Autodesk Inventor part; units mm, degrees
ref_plane "YZ Plane" through (0, 0, 0) normal (1, 0, 0) x (0, 1, 0)
ref_plane "XZ Plane" through (0, 0, 0) normal (0, 1, 0) x (-1, 0, 0)
ref_plane "XY Plane" through (0, 0, 0) normal (0, 0, 1) x (1, 0, 0)
sketch "Sketch1" plane through (0, 0, 0) normal (0, 0, 1) x (1, 0, 0)
  circle A0 centre (0, 0) radius 558
  circle A1 centre (0, 0) radius 580
  line L0 (0, 0) -> (-580, 0)
  line L1 (0, 0) -> (0, 580) construction
  line L2 (0, 0) -> (0, 580)
  circle A2 centre (0, 0) radius 100
  line L3 (197.082, 197.082) -> (278.716, 0)
  line L4 (278.716, 0) -> (197.082, -197.082)
  line L5 (197.082, -197.082) -> (0, -278.716)
  line L6 (0, -278.716) -> (-197.082, -197.082)
  line L7 (-197.082, -197.082) -> (-278.716, 0)
  line L8 (-278.716, 0) -> (-197.082, 197.082)
  line L9 (-197.082, 197.082) -> (0, 278.716)
  line L10 (0, 278.716) -> (197.082, 197.082)
  point P0 (-558, 0)
  point P1 (0, 558)
  point P2 (-100, 0)
  point P3 (0, 100)
  point P4 (0, 278.716)
  point P5 (-278.716, 0)
  dimension "d30" = 90
  dimension "d31" = 1160
  dimension "d32" = 1116
  dimension "d65" = 90
  dimension "d66" = 200
  dimension "d91" = 515
extrude "Plate1" add sketch "Sketch1" against normal blind 3 contours A0 L0 A1 L2 picked at (-572.0249, 22.0563)
sketch "Sketch2" plane through (0, 0, 0) normal (0, 0, 1) x (1, 0, 0)
  circle A0 centre (0, 0) radius 567.5
  arc A1 (0, 580) -> (-580, 0) centre (0, 0) ccw
  line L0 (0, 0) -> (0, 580) construction
  line L1 (0, 0) -> (-18.5681, 567.1962) construction
  line L2 (-128.8658, 552.6752) -> (0, 0) construction
  line L3 (0, 0) -> (0, 567.5) construction
  line L4 (0, 0) -> (18.5681, 567.1962) construction
  line L5 (0, 0) -> (128.8658, 552.6752) construction
  line L6 (0, 0) -> (-164.7366, 543.0636) construction
  line L7 (0, 0) -> (-267.5176, 500.4903) construction
  dimension "d34" = 1135
  dimension "d35" = 1.875
  dimension "d36" = 11.25
  dimension "d44" = 1.875
  dimension "d45" = 11.25
  dimension "d49" = 3.75
  dimension "d50" = 11.25
hole "Hole1" at (-18.5681, 567.1962, 0) at (-128.8658, 552.6752, 0) at (128.8658, 552.6752, 0) at (18.5681, 567.1962, 0) at (-164.7366, 543.0636, 0) at (-267.5176, 500.4903, 0) direction (0, 0, -1) diameter 8 end through all
pattern_circular "Circular Pattern1" count 4 over 90 about axis through (0, 0, -10) along (0, 0, 1) of "Hole1"
equation "\"d31\" = Колесо_диам1_ручья_внеш"
equation "\"d91\" = Барабан_размер_по_плоскостям"
equation "\"d44\" = d35"
equation "\"d45\" = d36"
equation "\"d49\" = 2 * d35"
equation "\"d50\" = d36"
equation "\"d42\" = Thickness"
equation "\"d15\" = Thickness"
equation "\"BendRadius\" = Thickness"
equation "\"BendReliefWidth\" = Thickness"
equation "\"BendReliefDepth\" = 0.5 * Thickness"
equation "\"CornerReliefSize\" = 4 * Thickness"
equation "\"MinimumRemnant\" = 2 * Thickness"
equation "\"TransitionRadius\" = BendRadius"
equation "\"JacobiRadiusSize\" = BendRadius"
equation "\"GapSize\" = Thickness"
properties part number "DMF 2.1 01 43 Gear rim 3_CPY" material "Stainless Steel"
Geometry: final body of the model. Coordinates: model frame, mm. Round coordinates to 2 decimals unless told otherwise and drop trailing zeros. Order: outer loops, then holes, each group sorted by start corner. A loop starts at its lowest first (then second) coordinate and runs counter-clockwise, first axis right, second up. Notation, with made-up numbers: M 10,66 L 34,66 A35 cw 34,99 Z; hole C 55,63.25 d7. An arc over 180 degrees is marked long. Use one line per item in the form item = value. Start each with the question number.
Q1. Cut plane B-B (y = 205). Return loops of the section in (x, z).
Q2. Pin query (flat end, axial travel): pin 1 Ø5 at (x, y) = (-128.87, 552.68) entering from -Z; pin 2 Ø1.5 at (y, z) = (237, -0.5) entering from +X. Return the tip coordinate at first contact, or that it passes through.
Q3. Cut plane C-C (x = -253.5). Return loops of the section in (y, z).
Q4. Cut plane A-A (z = -1.15). Count the separate pieces of the cut face and the enclosed holes in it, and give its area (3 significant figures).
Q5. Material intervals for line 1 (Y direction, x = -301, z = -2.1); line 2 (X direction, y = 167.5, z = -0.05); line 3 (Y direction, x = -93, z = -1.3), sorted ascending. Write a range as [from, to].
Geometry results:
q1.outline = M -542.56,-3 L -518.98,-3 L -518.98,0 L -542.56,0 Z
q2.pin_1 = through
q2.pin_2 = -504.82
q3.outline = M 497.09,-3 L 521.67,-3 L 521.67,0 L 497.09,0 Z
q4.separate_pieces = 1
q4.enclosed_holes = 12
q4.area = 19,100 mm^2
q5.line_1 = [469.85, 478.15], [485.7, 495.78]
q5.line_2 = [-555.29, -545.96], [-540.17, -532.27]
q5.line_3 = [550.2, 572.5]
